Model file for the job. Use its own axes, mm. Give positions to 0.01 mm unless a question says otherwise; leave off trailing zeros. Loops run counter-clockwise (first coordinate to the right, second up) from the corner with the lowest first, then second, coordinate; pieces in that order, holes last. Notation, with made-up numbers: M 70.25,5.5 L 115.25,5.5 A26 cw 115.25,28.5 Z; hole C -33,87 d5. An arc over 180 degrees is marked long. Answer in a Markdown table with one row per item.
```python
from build123d import *

# Parameters (mm, degrees)
SKETCH1_R           = 6.35
BOSS_EXTRUDE1_DEPTH = 38.1


with BuildPart() as part:
    # Sketch1 → Boss-Extrude1 (new body)
    with BuildSketch(Plane(origin=(0, 0, 0), x_dir=(1, 0, 0), z_dir=(0, 1, 0))):
        with BuildLine():
            Line((0, 0), (-292.1, 0))
            ThreePointArc((-292.1, 0), (-301.080256121, 3.719743879), (-304.8, 12.7))
            Line((-304.8, 12.7), (-304.8, 38.1))
            ThreePointArc((-304.8, 38.1), (-301.080256121, 47.080256121), (-292.1, 50.8))
            Line((-292.1, 50.8), (0, 50.8))
            Line((0, 50.8), (0, 0))
        make_face()
        with Locations(Location((-285.75, 25.4, 0), (0, 0, 90))):
            Circle(SKETCH1_R, mode=Mode.SUBTRACT)
    extrude(amount=BOSS_EXTRUDE1_DEPTH)


solid = part.part
```
Q1. Mould opens along Z. For faces 1 (the face through (-304.8, 19, -25)), 2 (the face through (-144, 19, 0)), 3 (the face through (-292.046, 18.783, -24.573)) say: released by +Z, released by -Z, zero draft, split by the parting line, or undercut.
Reported:
| item | result |
|---|---|
| face 1 | zero draft |
| face 2 | released by +Z |
| face 3 | undercut |
Q2. Saw through at A-A (x = -285.75). Give the cut face in (y, z), and give its area (3 significant figures).
Reported:
| item | result |
|---|---|
| outline | M 0,-50.8 L 38.1,-50.8 L 38.1,-31.75 L 0,-31.75 Z; M 0,-19.05 L 38.1,-19.05 L 38.1,0 L 0,0 Z |
| area | 1,450 mm² |
Q3. Probe probe 1 along Z at (x, y) = (-285.75, 29); probe 2 along X at (y, z) = (16, -25.4); probe 3 along X at (y, z) = (19.5, -27.5). List the from-to ranges inside material, lowest first.
Reported:
| item | result |
|---|---|
| probe 1 | -50.8 to -31.75, -19.05 to 0 |
| probe 2 | -304.8 to -292.1, -279.4 to 0 |
| probe 3 | -304.8 to -291.74, -279.76 to 0 |
Q4. Saw through at B-B (z = -25.4). Give the cut face in (x, y).
Reported:
| item | result |
|---|---|
| outline | M -304.8,0 L -292.1,0 L -292.1,38.1 L -304.8,38.1 Z; M -279.4,0 L 0,0 L 0,38.1 L -279.4,38.1 Z |
